Work out the finished part from the listing and answer in its coordinate system (mm). Coordinates: 2 decimals unless noted, no trailing zeros. Loops run counter-clockwise (first coordinate to the right, second up) from the corner with the lowest first, then second, coordinate; pieces in that order, holes last. Notation, with made-up numbers: (25, 53.5) -> (60, 53.5) arc R25 ccw to (60, 82.5) -> close; hole circle Ø4 at (4.25, 81.25). An arc over 180 degrees is marked (long way). Use a Markdown table: item, result.
from build123d import *

# Parameters (mm, degrees)
CROQUIS1_R              = 5
SALIENTE_EXTRUIR1_DEPTH = 5
REDONDEO1_R             = 5


with BuildPart() as part:
    # Croquis1 → Saliente-Extruir1 (new body)
    with BuildSketch(Plane(origin=(0, 0, 0), x_dir=(1, 0, 0), z_dir=(0, 1, 0))):
        Polygon((0, 0), (119.999982993, 2), (119.999982993, 16), (0, 18), align=None)
        with Locations(Location((10, 9, 0), (0, 0, 270))):
            Circle(CROQUIS1_R, mode=Mode.SUBTRACT)
        with Locations(Location((110, 9, 0), (0, 0, 270))):
            Circle(CROQUIS1_R, mode=Mode.SUBTRACT)
    extrude(amount=SALIENTE_EXTRUIR1_DEPTH)

    # Redondeo1
    redondeo1_edges = [part.edges().sort_by_distance(p)[0] for p in [
        (0, 2.5, -18),
        (119.999982993, 2.5, -16),
        (119.999982993, 2.5, -2),
        (0, 2.5, 0),
    ]]
    fillet(redondeo1_edges, radius=REDONDEO1_R)


solid = part.part
Q1. Section B-B on y = 4.2 is taken. Determine the outline of the cut face in (x, z).
Solved:
| item | result |
|---|---|
| outline | (0, -12.92) arc R5 ccw to (5.08, -17.92) -> (115.08, -16.08) arc R5 ccw to (120, -11.08) -> (120, -6.92) arc R5 ccw to (115.08, -1.92) -> (5.08, -0.08) arc R5 ccw to (0, -5.08) -> close; hole circle Ø10 at (10, -9); hole circle Ø10 at (110, -9) |
Q2. Section C-C on x = 110 is taken. Determine the outline of the cut face in (y, z).
Solved:
| item | result |
|---|---|
| outline | (0, -16.17) -> (5, -16.17) -> (5, -14) -> (0, -14) -> close; (0, -4) -> (5, -4) -> (5, -1.83) -> (0, -1.83) -> close |
Q3. Given pin 1 Ø2 at (x, y) = (41.5, 3.5) entering from +Z (3 decimals); pin 2 Ø1.5 at (y, z) = (1.5, -2) entering from +X, each flat-ended and moving along its own axis, determine where each tip first touches the part or whether it passes through.
Solved:
| item | result |
|---|---|
| pin 1 | z = -0.675 |
| pin 2 | x = 117.76 |
Q4. Consider line 1 (X direction, y = 3.2, z = -9); line 2 (X direction, y = 2.1, z = -7.5); line 3 (Z direction, x = 6, y = 1.6). Determine where each line is inside the solid, lowest interval first. Write a range as [from, to].
Solved:
| item | result |
|---|---|
| line 1 | [0, 5], [15, 105], [115, 120] |
| line 2 | [0, 5.23], [14.77, 105.23], [114.77, 120] |
| line 3 | [-17.9, -12], [-6, -0.1] |
Q5. Determine the mould class of faces 1 (the cylindrical face through (118.527, 2.535, -3.373)), 2 (the cylindrical face through (11.5, 2.46, -4.23)), 3 (the flat face through (59, 5, -9)) for opening direction Z: pulls with the +Z half, pulls with the -Z half, needs draft (parallel to the pull), parting line crosses it, or undercut.
Solved:
| item | result |
|---|---|
| face 1 | pulls with the +Z half |
| face 2 | undercut |
| face 3 | needs draft |
Q6. Section A-A on z = -9 is taken. Determine the outline of the cut face in (x, y), and give its area (3 significant figures).
Solved:
| item | result |
|---|---|
| outline | (0, 0) -> (5, 0) -> (5, 5) -> (0, 5) -> close; (15, 0) -> (105, 0) -> (105, 5) -> (15, 5) -> close; (115, 0) -> (120, 0) -> (120, 5) -> (115, 5) -> close |
| area | 500 mm² |
Q7. Section D-D on x = 10 is taken. Determine the outline of the cut face in (y, z).
Solved:
| item | result |
|---|---|
| outline | (0, -17.83) -> (5, -17.83) -> (5, -14) -> (0, -14) -> close; (0, -4) -> (5, -4) -> (5, -0.17) -> (0, -0.17) -> close |
